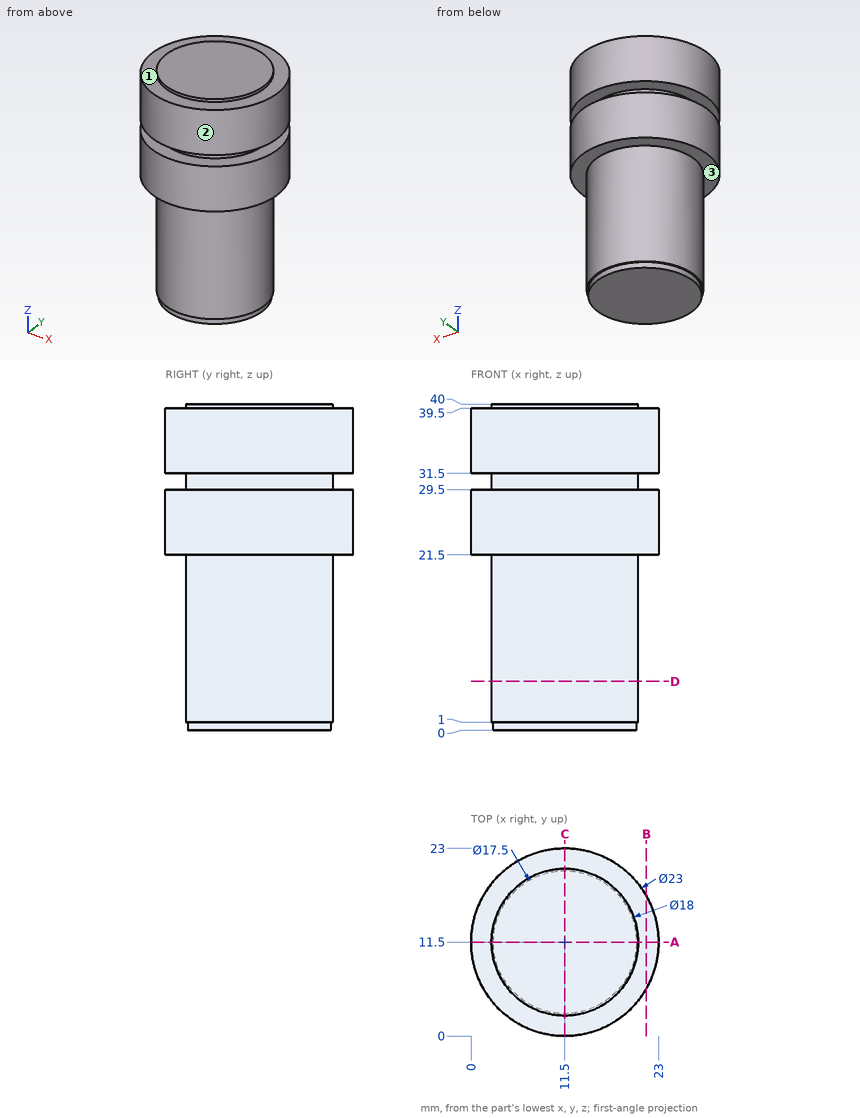
Drawing for the job (mm, zero at the part's lowest x, y, z). A direction names the side the tool comes from. Coordinates: 2 decimals unless noted, no trailing zeros. Order: outer loops, then holes, each group sorted by start corner. A loop starts at its lowest first (then second) coordinate and runs counter-clockwise, first axis right, second up. Notation, with made-up numbers: (0.5, -27.75) -> (34.5, -27.75) arc R21 ccw to (34.5, -12.75) -> close; hole circle Ø1 at (-39.5, 43). An arc over 180 degrees is marked (long way). Return JSON: item names as keys, results as strings.
Item 1: Slice it at D-D (z = 6). Write the cut outline in (x, y), then the cut area to 3 significant figures.
Model answer:
{"outline": "circle Ø18 at (11.5, 11.5)", "area": "254 mm²"}
Item 2: Slice it at A-A (y = 11.5). Write the cut outline in (x, z), then the cut area to 4 significant figures.
Model answer:
{"outline": "(0, 21.5) -> (2.5, 21.5) -> (2.5, 1) -> (2.75, 1) -> (2.75, 0) -> (20.25, 0) -> (20.25, 1) -> (20.5, 1) -> (20.5, 21.5) -> (23, 21.5) -> (23, 29.5) -> (20.5, 29.5) -> (20.5, 31.5) -> (23, 31.5) -> (23, 39.5) -> (20.5, 39.5) -> (20.5, 40) -> (2.5, 40) -> (2.5, 39.5) -> (0, 39.5) -> (0, 31.5) -> (2.5, 31.5) -> (2.5, 29.5) -> (0, 29.5) -> close", "area": "799.5 mm²"}
Item 3: Wall check: line 1 along Z through (x, y) = (21, 7.25); line 2 along Y through (x, z) = (6, 20); line 3 along X through (y, z) = (16, 8). Give the ranges that are in metal, low to high. Write a range as from..to.
Model answer:
{"line 1": "z = 21.5..29.5, 31.5..39.5", "line 2": "y = 4.38..18.62", "line 3": "x = 3.71..19.29"}
Item 4: Pin check, flat tips, straight feed: P1, Ø1, axis at x = 19, z = 16.5, coming from the +Y side; P2, Ø5, axis at y = 13, z = 13, coming from the +X side; P3, Ø5, axis at y = 7, z = 14.5, coming from the +X side. Stop position of each tip, or through.
Model answer:
{"P1": "stops at y = 17.16", "P2": "stops at x = 20.5", "P3": "stops at x = 20.27"}
Item 5: 3-axis set-ups, long thin cutter, end or side, ignore diameter. For the marked faces 1, 2 and 3: which of +Z, -Z, +X, -X, +Y, -Y reach the whole face in a straight line?
Model answer:
{"face 1": "+Z", "face 2": "+Z, -Z", "face 3": "-Z"}
Item 6: Slice it at B-B (x = 21.5). Write the cut outline in (y, z).
Model answer:
{"outline": "(5.82, 21.5) -> (17.18, 21.5) -> (17.18, 29.5) -> (5.82, 29.5) -> close; (5.82, 31.5) -> (17.18, 31.5) -> (17.18, 39.5) -> (5.82, 39.5) -> close"}
